The listing builds one solid part. Answer for the finished solid, in the listing's coordinates (mm). A direction names the side the tool comes from. Coordinates: 2 decimals unless noted, no trailing zeros. Order: outer loops, then holes, each group sorted by start corner. A loop starts at its lowest first (then second) coordinate and runs counter-clockwise, first axis right, second up. Notation, with made-up numbers: (-11, 56) - (36, 56) arc R14 ccw to (36, 76) - close; hole circle Ø5 at (22, -28.5). An arc over 180 degrees is marked (long way). One line per item, written item: value. Start each with the question number.
```python
from build123d import *

# Parameters (mm, degrees)
SKETCH1_R           = 9.525
SKETCH1_R_2         = 2.3495
EXTRUDE1_DEPTH      = 24.78278
SKETCH2_OUTSIDE_W   = 28.372
SKETCH2_OUTSIDE_H   = 28.372
SKETCH2_OUTSIDE_R   = 5.1562
EXTRUDE2_DEPTH      = 6.096
EXTRUDE3_DEPTH      = 29.207045831
EXTRUDE3_DEPTH_BACK = 29.207045831


with BuildPart() as part:
    # Sketch1 → Extrude1 (new body)
    with BuildSketch(Plane.XY):
        Circle(SKETCH1_R)
        Circle(SKETCH1_R_2, mode=Mode.SUBTRACT)
    extrude(amount=EXTRUDE1_DEPTH)

    # Sketch2 outside → Extrude2 (cut)
    with BuildSketch(Plane.XY.offset(18.48358)):
        Rectangle(SKETCH2_OUTSIDE_W, SKETCH2_OUTSIDE_H)
        Circle(SKETCH2_OUTSIDE_R, mode=Mode.SUBTRACT)
    extrude(amount=-EXTRUDE2_DEPTH, mode=Mode.SUBTRACT)

    # Sketch3 → Extrude3 (cut, two sides: drawn at the far end of the back side and taken through both)
    with BuildSketch(Plane(origin=(0, 0, 0), x_dir=(1, 0, 0), z_dir=(0, 1, 0)).offset(-EXTRUDE3_DEPTH_BACK)):
        with BuildLine():
            Line((81.364445057, 9.888659405), (9.525, 0))
            ThreePointArc((9.525, 0), (0, -0.652479271), (-9.525, 0))
            Line((-9.525, 0), (-81.364445057, 9.888659405))
            Line((-81.364445057, 9.888659405), (-81.364445057, 154.92233068))
            Line((-81.364445057, 154.92233068), (81.364445057, 154.92233068))
            Line((81.364445057, 154.92233068), (81.364445057, 9.888659405))
        make_face()
    extrude(amount=EXTRUDE3_DEPTH + EXTRUDE3_DEPTH_BACK, mode=Mode.SUBTRACT)


solid = part.part
```
(1) Consider probe 1 along Y at (x, z) = (0, 19.5) (1 decimal); probe 2 along Y at (x, z) = (0, 17.5). Determine where each line is inside the solid, lowest interval first.
(2) The part is cut by section B-B on z = 15. Determine the outline of the cut face in (x, y), plus the area to 3 significant figures.
(3) For faces 1 (the face through (4, -4, 12.388)), 2 (the face through (-7.559, -5.796, 21.589)), determine the directions among +Z, -Z, +X, -X, +Y, -Y from which every point of the face is accessible in a straight line to the end or side of a thin tool.
(4) The part is cut by section A-A on x = 0. Determine the outline of the cut face in (y, z) (1 decimal), plus the area to 3 significant figures.
(5) Flat-ended cylindrical pins translate along their axes: pin 1 Ø1.5 at (x, z) = (-2.5, 19.5) entering from +Y; pin 2 Ø1 at (x, z) = (-1, 14) entering from +Y; pin 3 Ø3 at (x, z) = (-4.5, 10.5) entering from +Y. Find the tip coordinate at first contact, or state that the pin passes through.
(6) For a pull along Y with two mould halves and no side action, classify faces 3 (the face through (-0.31, 2.33, 12.53)), 4 (the face through (4, -4, 18.484)), 5 (the face through (9.085, 2.861, 6.107)) as pulls with the +Y half, pulls with the -Y half, needs draft (parallel to the pull), parting line crosses it, or undercut.
Completed:
1. probe 1: y = -9.5 to -2.3, 2.3 to 9.5
1. probe 2: y = -5.16 to -2.35, 2.35 to 5.16
2. outline: circle Ø10.31 at (0, 0); hole circle Ø4.7 at (0, 0)
2. area: 66.2 mm2
3. face 1: none
3. face 2: +Z, -Z
4. outline: (-9.5, 0.7) - (-2.3, 0.7) - (-2.3, 24.8) - (-9.5, 24.8) - (-9.5, 18.5) - (-5.2, 18.5) - (-5.2, 12.4) - (-9.5, 12.4) - close; (2.3, 0.7) - (9.5, 0.7) - (9.5, 12.4) - (5.2, 12.4) - (5.2, 18.5) - (9.5, 18.5) - (9.5, 24.8) - (2.3, 24.8) - close
4. area: 293 mm2
5. pin 1: stops at y = 9.36
5. pin 2: stops at y = 5.13
5. pin 3: stops at y = 9.04
6. face 3: undercut
6. face 4: needs draft
6. face 5: parting line crosses it
